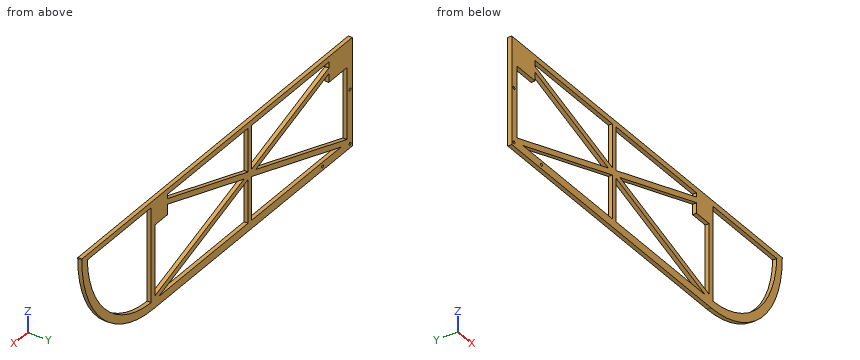
```python
from build123d import *

# Parameters (mm, degrees)
SKETCH_1_R          = 1
EXTRUDE_1_DEPTH     = 3
CUT_EXTRUDE_2_DEPTH = 18


with BuildPart() as part:
    # 草图1 → 凸台-拉伸1 (new body)
    with BuildSketch(Plane(origin=(0, 0, 0), x_dir=(1, 0, 0), z_dir=(0, 1, 0))):
        with BuildLine():
            Line((-150, 40), (71, 40))
            ThreePointArc((71, 40), (126.861435714, 16.861435714), (150, -39))
            Line((150, -39), (150, -40))
            Line((150, -40), (-150, -40))
            Line((-150, -40), (-150, 40))
        make_face()
        with Locations(Location((-117.057778193, 37, 0), (0, 0, 270))):
            Circle(SKETCH_1_R, mode=Mode.SUBTRACT)
        with Locations(Location((-147.557778193, 37, 0), (0, 0, 270))):
            Circle(SKETCH_1_R, mode=Mode.SUBTRACT)
        with Locations(Location((-147.557778193, -3, 0), (0, 0, 270))):
            Circle(SKETCH_1_R, mode=Mode.SUBTRACT)
    extrude(amount=EXTRUDE_1_DEPTH)

    # 草图4 → 切除-拉伸2 (cut)
    with BuildSketch(Plane(origin=(0, 0, 0), x_dir=(1, 0, 0), z_dir=(0, 1, 0))):
        with BuildLine():
            ThreePointArc((143.938330115, -36), (122.26382188, 12.971343703), (73, 33.972597597))
            Line((73, 33.972597597), (73, -36))
            Line((73, -36), (143.938330115, -36))
        make_face()
        Polygon((-34.5, 1.754496568), (64.53976054, 34), (-34.5, 34), align=None)
        Polygon((69, -21), (69, 31.245503432), (-30.03976054, -1), (55, -28.687363897), (55, -21), align=None)
        Polygon((-38.5, 1.754496568), (-38.5, 34), (-137.53976054, 34), align=None)
        Polygon((55, -36), (55, -32.894031452), (-34.5, -3.754496568), (-34.5, -36), align=None)
        Polygon((-124, -27.385038315), (-42.96023946, -1), (-144, 31.896666222), (-144, -21), (-124, -21), align=None)
        Polygon((-38.5, -36), (-38.5, -3.754496568), (-124, -31.591705871), (-124, -36), align=None)
    extrude(amount=CUT_EXTRUDE_2_DEPTH, mode=Mode.SUBTRACT)


solid = part.part
```
The model under review builds one solid part; all positions refer to its coordinate system, in mm. Give positions to 0.01 mm unless a question says otherwise; leave off trailing zeros. Write each loop counter-clockwise with the first axis right and the second up, starting at its lowest first coordinate (ties: lowest second). Pieces come first, ordered by that corner, then holes.
(1) For P1, Ø1.2, axis at x = -147.56, z = -37, coming from the -Y side; P2, Ø1.5, axis at y = 1, z = 24, coming from the +X side; P3, Ø0.9, axis at y = 1.5, z = 16.5, coming from the +X side; P4, Ø1.5, axis at y = 1, z = -17.5, coming from the +X side, all flat-tipped, find the tip position at first contact; note any pin that passes through.
(2) Consider section C-C, the plane x = -130. Give the boundary of the cut face in (y, z).
(3) To check wall thickness, follow L1, parallel to X at y = 0.8, z = 35; L2, parallel to Z at x = -129, y = 0.7; L3, parallel to Z at x = -137, y = 1.1. State the ranges of each line that lie inside material, in increasing order.
(4) Consider section A-A, the plane x = -80. Give the boundary of the cut face in (y, z).
(5) Consider section D-D, the plane z = 18.5. Give the boundary of the cut face in (x, y), and give its area (3 significant figures).
(6) Consider section B-B, the plane z = -16. Give the boundary of the cut face in (x, y).
Returned:
1. P1: passes through
1. P2: stops at x = 148.7
1. P3: stops at x = 146.86
1. P4: stops at x = 126.97
2. outline: (0, -40) - (3, -40) - (3, -34) - (0, -34) - close; (0, -31.55) - (3, -31.55) - (3, -27.34) - (0, -27.34) - close; (0, 21) - (3, 21) - (3, 40) - (0, 40) - close
3. L1: x = -150 to -124, -38.5 to -34.5, 55 to 73, 143.89 to 149.9
3. L2: z = -40 to -34, -31.22 to -27.01, 21 to 40
3. L3: z = -40 to -34, -33.82 to -29.62, 21 to 40
4. outline: (0, -40) - (3, -40) - (3, -34) - (0, -34) - close; (0, -15.27) - (3, -15.27) - (3, -11.06) - (0, -11.06) - close; (0, 13.06) - (3, 13.06) - (3, 17.27) - (0, 17.27) - close; (0, 36) - (3, 36) - (3, 40) - (0, 40) - close
5. outline: (-150, 0) - (-144, 0) - (-144, 3) - (-150, 3) - close; (-96.71, 0) - (-83.79, 0) - (-83.79, 3) - (-96.71, 3) - close; (-38.5, 0) - (-34.5, 0) - (-34.5, 3) - (-38.5, 3) - close; (10.79, 0) - (23.71, 0) - (23.71, 3) - (10.79, 3) - close; (69, 0) - (73, 0) - (73, 3) - (69, 3) - close; (141.06, 0) - (147.29, 0) - (147.29, 3) - (141.06, 3) - close
5. area: 138 mm2
6. outline: (-150, 0) - (-144, 0) - (-144, 3) - (-150, 3) - close; (-95.17, 0) - (-82.25, 0) - (-82.25, 3) - (-95.17, 3) - close; (-38.5, 0) - (-34.5, 0) - (-34.5, 3) - (-38.5, 3) - close; (9.25, 0) - (22.17, 0) - (22.17, 3) - (9.25, 3) - close; (69, 0) - (73, 0) - (73, 3) - (69, 3) - close; (119, 0) - (127.71, 0) - (127.71, 3) - (119, 3) - close
